Autodesk Inventor part; units mm, degrees
ref_plane "YZ Plane" through (0, 0, 0) normal (1, 0, 0) x (0, 1, 0)
ref_plane "XZ Plane" through (0, 0, 0) normal (0, 1, 0) x (-1, 0, 0)
ref_plane "XY Plane" through (0, 0, 0) normal (0, 0, 1) x (1, 0, 0)
sketch "Sketch1" plane through (0, 0, 0) normal (0, 0, 1) x (1, 0, 0)
  line L0 (0, 0) -> (0, 12.7)
  line L1 (0, 5.5563) -> (5.5562, 5.5563)
  line L2 (0, 7.9375) -> (26.1937, 7.9375)
  line L3 (26.1937, 7.9375) -> (26.1937, 5.5563)
  line L4 (26.1937, 5.5563) -> (26.1937, 0)
  line L5 (26.1937, 0) -> (0, 0)
  line L6 (26.1938, 6.35) -> (34.3852, 6.35)
  line L7 (26.1937, 0) -> (34.3852, 0)
  line L8 (34.3852, 0) -> (34.3852, 6.35)
  line L9 (16.6687, 7.9375) -> (16.6687, 0)
  circle A0 centre (16.6687, 7.5565) radius 2.3813
  circle A1 centre (16.6687, 5.4928) radius 2.3813
  circle A2 centre (10.3187, 7.5565) radius 2.3813
  circle A3 centre (10.3187, 5.4928) radius 2.3813
  line L10 (10.3187, 7.9375) -> (10.3187, 0)
  line L11 (0, 5.1753) -> (26.1938, 5.1753)
  line L12 (8.7312, 5.1753) -> (8.7312, 0)
  line L13 (5.5562, 5.1753) -> (5.5562, 3.3734)
  line L14 (18.2562, 5.1753) -> (18.2562, 0)
  line L15 (21.4312, 5.1753) -> (21.4312, 0)
  line L16 (0, 3.1115) -> (26.1937, 3.1115)
  line L17 (5.5562, 3.1115) -> (8.7312, 5.1753)
  line L18 (18.2562, 5.1753) -> (21.4312, 3.1115)
  line L19 (11.9062, 5.1753) -> (11.9062, 0)
  line L20 (15.0812, 5.1753) -> (15.0812, 0)
  line L21 (11.9062, 5.1753) -> (15.0812, 3.1115)
  line L22 (21.4312, 3.3734) -> (34.3852, 3.3734)
  line L23 (24.6062, 3.3734) -> (24.6062, 0)
  line L24 (21.4312, 3.3734) -> (20.1197, 5.5563)
  line L25 (26.1937, 3.1115) -> (30.9563, 3.1115)
  line L26 (30.9563, 3.1115) -> (30.9563, 0)
  line L27 (31.75, 3.3734) -> (31.75, 0)
  line L28 (31.75, 0) -> (29.723, 3.3734)
  line L29 (0, 7.9375) -> (-8.7312, 7.9375)
  line L30 (0, 3.3734) -> (5.5562, 3.3734)
  line L31 (5.5562, 5.1753) -> (5.5562, 5.5563)
  line L32 (5.5562, 5.5563) -> (26.1937, 5.5563)
  line L33 (0, 5.5563) -> (-8.7312, 5.5562)
  line L34 (-10.3187, 7.9375) -> (-10.3187, 3.3734)
  line L35 (-10.3187, 3.3734) -> (0, 3.3734)
  line L36 (-8.7312, 7.9375) -> (-8.7312, 5.5562)
  line L37 (-8.7312, 7.9375) -> (-10.3187, 7.9375)
  line L38 (5.5562, 3.3734) -> (5.5562, 0)
  dimension "d0" = 12.7
  dimension "d1" = 5.5563
  dimension "d2" = 7.9375
  dimension "d3" = 26.1938
  dimension "d4" = 8.1915
  dimension "d5" = 6.35
  dimension "d6" = 9.525
  dimension "d7" = 6.35
  dimension "d8" = 0.381
  dimension "d9" = 0.381
  dimension "d10" = 0.0635
  dimension "d11" = 0.0635
  dimension "d12" = 1.5875
  dimension "d13" = 4.7625
  dimension "d14" = 1.5875
  dimension "d15" = 4.7625
  dimension "d16" = 3.1115
  dimension "d17" = 1.5875
  dimension "d18" = 4.7625
  dimension "d19" = 3.3734
  dimension "d20" = 3.175
  dimension "d21" = 31
  dimension "d22" = 9.525
  dimension "d23" = 9.525
  dimension "d24" = 0.7937
  dimension "d25" = 31
  dimension "d27" = 3.3734
  dimension "d33" = 4.7625
  dimension "d34" = 8.7312
  dimension "d35" = 1.5875
revolve "Revolution1" add sketch "Sketch1" angle 360 about axis through (26.1937, 0, 0) along (-1, 0, 0) contours L35 L34 L37 L36 L33 L0 | L0 L11 L13 L30 | L0 L1 L31 L11
equation "\"d1\" = d28"
equation "\"d2\" = d29"
equation "\"d8\" = d30"
equation "\"d9\" = d8"
equation "\"d10\" = d31"
equation "\"d11\" = d10"
equation "\"d16\" = d32"
equation "\"d17\" = d12"
equation "\"d18\" = d13"
equation "\"d23\" = d22"
equation "\"d25\" = d21"
equation "\"d27\" = d19"
properties part number "Output Shaft Insert"
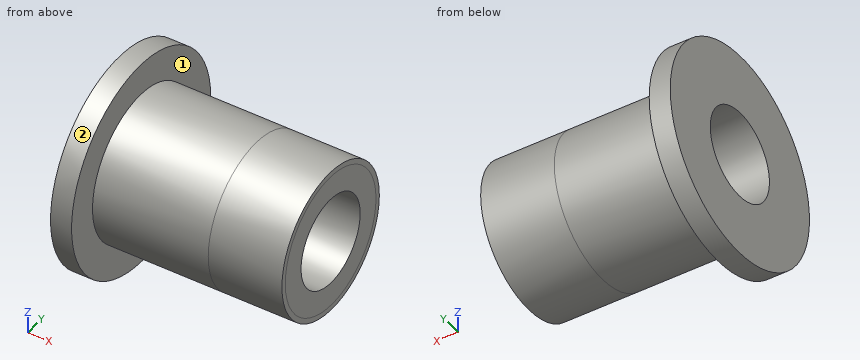
Build history of the part. All positions in model axes, mm. Face numbers are marked on the shaded views. A direction names the side the tool comes from. Give positions to 0.01 mm unless a question says otherwise; leave off trailing zeros. Loops run counter-clockwise (first coordinate to the right, second up) from the corner with the lowest first, then second, coordinate; pieces in that order, holes last. Notation, with made-up numbers: (-39, 71.5) - (6, 71.5) arc R31 cw to (6, 106.5) - close; hole circle Ø7 at (47.5, -23). An arc over 180 degrees is marked (long way). Write item = value, one per line. Start each with the question number.
1) Band-saw the part on D-D on y = 4.75. Give the cut face in (x, z).
2) Band-saw the part on C-C on x = -9.25. Give the cut face in (y, z) (1 decimal).
3) Band-saw the part on A-A on z = -2.5. Give the cut face in (x, y), plus the area to 3 significant figures.
4) Tool access for the marked faces 1 and 2: list every direction of +Z, -Z, +X, -X, +Y, -Y with a clear straight run to the whole face (end or side of a thin tool).
5) Probe probe 1 along Y at (x, z) = (2.9, 0); probe 2 along Y at (x, z) = (3.75, -1). List the from-to ranges inside material, lowest first. Write a range as from..to.
6) Band-saw the part on B-B on y = 0. Give the cut face in (x, z), plus the area to 3 significant figures.
7) Drop flat-ended pins along their axis: pin 1 Ø4 at (x, z) = (-0.5, -1) entering from -Y; pin 2 Ø4 at (x, y) = (3, -4.5) entering from +Z; pin 3 Ø8 at (y, z) = (0, 0) entering from -X; pin 4 Ø6 at (x, y) = (-8.5, 4) entering from +Z. Give the stop position or say it passes through.
Final values:
q1.outline = (-10.32, -6.36) - (-8.73, -6.36) - (-8.73, -2.88) - (5.56, -2.88) - (5.56, 2.88) - (-8.73, 2.88) - (-8.73, 6.36) - (-10.32, 6.36) - close
q2.outline = circle Ø15.9 at (0, 0); hole circle Ø6.7 at (0, 0)
q3.outline = (-10.32, -7.53) - (-8.73, -7.53) - (-8.73, -4.96) - (5.56, -4.96) - (5.56, -2.26) - (-10.32, -2.26) - close; (-10.32, 2.26) - (5.56, 2.26) - (5.56, 4.96) - (-8.73, 4.96) - (-8.73, 7.53) - (-10.32, 7.53) - close
q3.area = 93.8 mm²
q4.face_1 = +X
q4.face_2 = +X, -X
q5.probe_1 = -5.56..-3.37, 3.37..5.56
q5.probe_2 = -5.47..-3.22, 3.22..5.47
q6.outline = (-10.32, -7.94) - (-8.73, -7.94) - (-8.73, -5.56) - (5.56, -5.56) - (5.56, -3.37) - (-10.32, -3.37) - close; (-10.32, 3.37) - (5.56, 3.37) - (5.56, 5.56) - (-8.73, 5.56) - (-8.73, 7.94) - (-10.32, 7.94) - close
q6.area = 76.9 mm²
q7.pin_1 = -5.56
q7.pin_2 = 4.96
q7.pin_3 = -10.32
q7.pin_4 = 7.87
